Verification items for this drawing (mm, ordinates from the low corner). A direction names the side the tool comes from. Give positions to 0.01 mm unless a question says otherwise; leave off trailing zeros. Loops run counter-clockwise (first coordinate to the right, second up) from the corner with the lowest first, then second, coordinate; pieces in that order, holes last. Notation, with made-up numbers: (-19.5, 8.25) -> (-7.5, 8.25) arc R26 ccw to (-7.5, 44.25) -> close; hole circle Ø9 at (16.25, -9.5). An arc over 180 degrees is marked (long way). Answer as a JSON object with one key per item and string values.
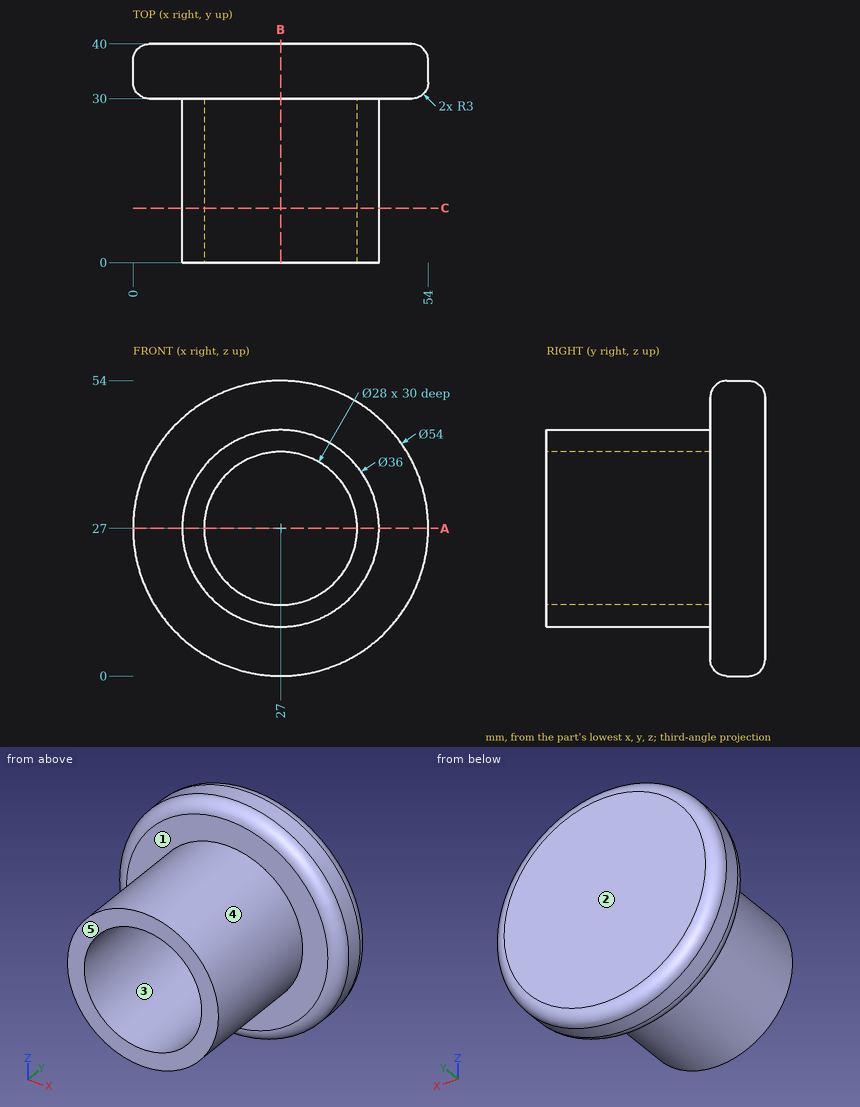
1) Depth check by flat-ended pin: P1, Ø1.5, axis at x = 29, y = 29.5, coming from the -Z side; P2, Ø5, axis at x = 19, y = 23, coming from the +Z side; P3, Ø1, axis at y = 25.5, z = 26.5, coming from the -X side. Enter the tip coordinate at first touch or a pass-through.
Geometry check:
{"P1": "stops at z = 1.88", "P2": "stops at z = 44.14", "P3": "stops at x = 9"}
2) Section check A-A on z = 27. Record the cut outline in (x, y).
Geometry check:
{"outline": "(0, 33) arc R3 ccw to (3, 30) -> (9, 30) -> (9, 0) -> (13, 0) -> (13, 30) -> (41, 30) -> (41, 0) -> (45, 0) -> (45, 30) -> (51, 30) arc R3 ccw to (54, 33) -> (54, 37) arc R3 ccw to (51, 40) -> (3, 40) arc R3 ccw to (0, 37) -> close"}
3) Draft check along X on the marked faces 3, 4 and 5. Enter one of: pulls with the +X half, pulls with the -X half, needs draft (parallel to the pull), parting line crosses it, or undercut.
Geometry check:
{"face 3": "undercut", "face 4": "parting line crosses it", "face 5": "needs draft"}
4) Tool access check on the marked faces 1 and 2. Record the directions out of +Z, -Z, +X, -X, +Y, -Y that give a thin tool (end or side, any length) a straight path to the whole face; none if there is none.
Geometry check:
{"face 1": "-Y", "face 2": "+Z, -Z, +X, -X, +Y"}
5) Material ranges on line 1 along Z through (x, y) = (27, 13.75); line 2 along Y through (x, z) = (40, 13); line 3 along X through (y, z) = (17, 19), recorded low to high. Write a range as from..to.
Geometry check:
{"line 1": "z = 9..13, 41..45", "line 2": "y = 30..40", "line 3": "x = 10.88..15.51, 38.49..43.12"}
6) Section check B-B on x = 27. Record the cut outline in (y, z).
Geometry check:
{"outline": "(0, 9) -> (30, 9) -> (30, 3) arc R3 ccw to (33, 0) -> (37, 0) arc R3 ccw to (40, 3) -> (40, 51) arc R3 ccw to (37, 54) -> (33, 54) arc R3 ccw to (30, 51) -> (30, 45) -> (0, 45) -> (0, 41) -> (30, 41) -> (30, 13) -> (0, 13) -> close"}
7) Section check C-C on y = 10. Record the cut outline in (x, z).
Geometry check:
{"outline": "circle Ø36 at (27, 27); hole circle Ø28 at (27, 27)"}
